Part print with two shaded views. Sizes in mm from the minimum x, y, z corner. A direction names the side the tool comes from. Give positions to 0.01 mm unless a question says otherwise; leave off trailing zeros. Write each loop counter-clockwise with the first axis right and the second up, starting at its lowest first coordinate (ties: lowest second). Pieces come first, ordered by that corner, then holes. Notation, with made-up numbers: M -33,62 L -5,62 A7 cw -5,74 Z; hole C 87.5,-31 d5. An arc over 180 degrees is marked long. Return JSON: item names as keys, results as strings. Group by question number.
Q1. Flat gauge pins, fed straight in: pin 1 Ø1.6 at (y, z) = (1, 42) entering from -X; pin 2 Ø1.5 at (x, y) = (87.5, 4.5) entering from -Z; pin 3 Ø1.6 at (y, z) = (0.5, 41) entering from +X; pin 4 Ø9.5 at (x, z) = (84, 67.5) entering from -Y. Where does each tip first touch, or does it go through?
Q2. Band-saw the part on C-C, the plane z = 59.5. Give the cut face in (x, y), then the cut area to 3 significant figures.
Q3. Wall check: probe 1 along X at (y, z) = (6, 80.5); probe 2 along X at (y, z) = (1.75, 92.5); probe 3 along Z at (x, y) = (92, 4.5). Give the ranges that are in metal, low to high.
Q4. Pull direction Z, two halves, no side cores. Call the marked faces 1, 2 and 3: +Z half, -Z half, draft (parallel to the pull), parting line (faces both ways), or undercut.
Q5. Band-saw the part on B-B, the plane x = 46. Give the cut face in (y, z), then the cut area to 3 significant figures.
Q6. Tool access for the marked faces 4 and 5: list every direction of +Z, -Z, +X, -X, +Y, -Y with a clear straight run to the whole face (end or side of a thin tool).
Q7. Band-saw the part on A-A, the plane y = 3.25. Give the cut face in (x, z).
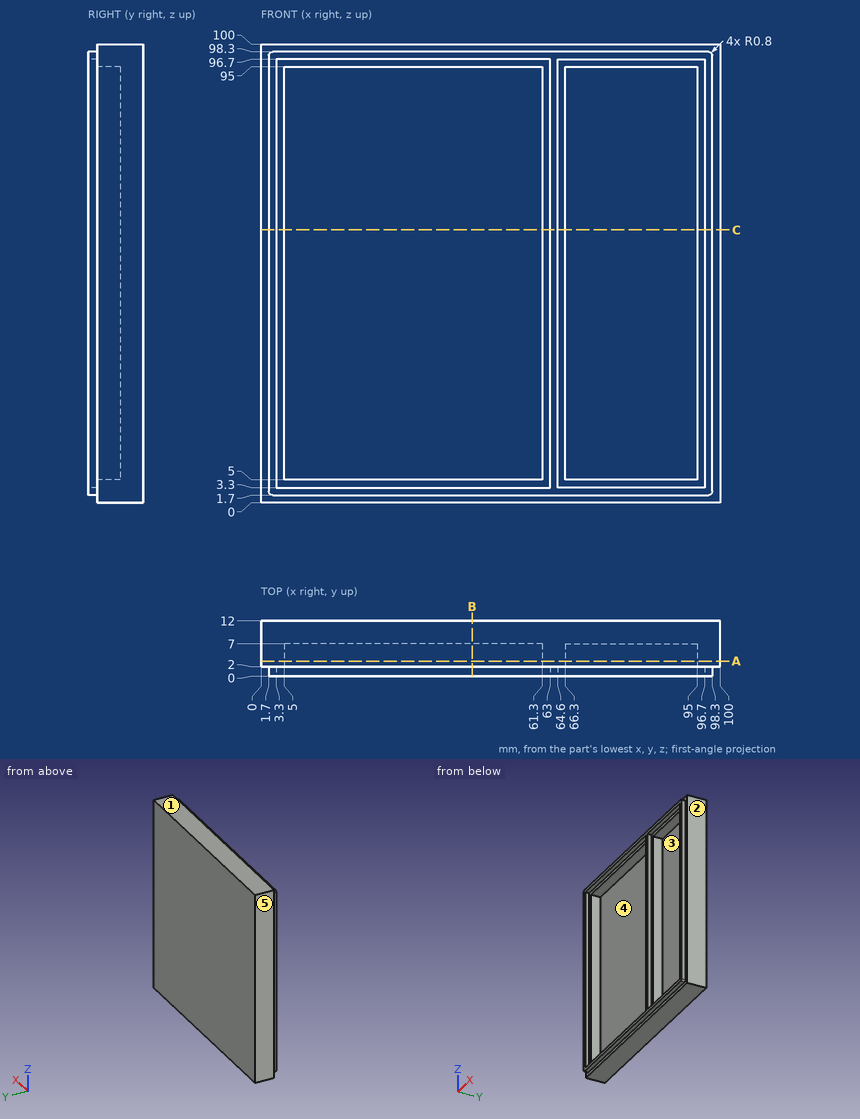
From the geometry:
{
 "1": {"pin 1": "stops at x = 1.7", "pin 2": "stops at z = 0", "pin 3": "stops at x = 98.3", "pin 4": "stops at y = 7"},
 "2": {"outline": "M 0,2 L 1.7,2 L 1.7,0 L 3.3,0 L 3.3,2 L 5,2 L 5,7 L 61.3,7 L 61.3,2 L 63,2 L 63,0 L 64.6,0 L 64.6,2 L 66.3,2 L 66.3,7 L 95,7 L 95,2 L 96.7,2 L 96.7,0 L 98.3,0 L 98.3,2 L 100,2 L 100,12 L 0,12 Z", "area": "585 mm^2"},
 "3": {"probe 1": "x = 0 to 5, 61.3 to 66.3, 95 to 100", "probe 2": "x = 1.7 to 3.3, 63 to 64.6, 96.7 to 98.3", "probe 3": "z = 0 to 5, 95 to 100"},
 "4": {"face 1": "+Z half", "face 2": "draft", "face 3": "undercut"},
 "5": {"outline": "M 0,1.7 L 2,1.7 L 2,0 L 12,0 L 12,100 L 2,100 L 2,98.3 L 0,98.3 L 0,96.7 L 2,96.7 L 2,95 L 7,95 L 7,5 L 2,5 L 2,3.3 L 0,3.3 Z", "area": "556 mm^2"},
 "6": {"face 4": "-Y", "face 5": "+Z, -Z, -X, +Y, -Y"},
 "7": {"outline": "M 0,0 L 100,0 L 100,100 L 0,100 Z; hole M 5,5 L 61.3,5 L 61.3,95 L 5,95 Z; hole M 66.3,5 L 95,5 L 95,95 L 66.3,95 Z"}
}
